Can you work these out from the model? Positions are in its coordinate system, mm. A direction names the side the tool comes from. Give positions to 0.01 mm unless a question says otherwise; leave off trailing zeros. Order: outer loops, then holes, each group sorted by start corner. A loop starts at its lowest first (then second) coordinate and runs counter-clockwise, first axis right, second up. Notation, with made-up numbers: (80, 52) - (129, 52) arc R22 cw to (129, 89) - close; hole circle Ø7 at (64, -15). An arc over 180 degrees is marked (long way). One line per question, with ' | ' between items.
```python
from build123d import *

# Parameters (mm, degrees)
SKETCH_1_R      = 1.5
EXTRUDE_1_DEPTH = 3


with BuildPart() as part:
    # 草图1 → 凸台-拉伸1 (new body)
    with BuildSketch(Plane.XY):
        with BuildLine():
            Line((-3, -336.18), (-3, -372.501331749))
            Line((-3, -372.501331749), (116, -372.501331749))
            Line((116, -372.501331749), (116, -336.18))
            ThreePointArc((116, -336.18), (118, -332.18), (116, -328.18))
            Line((116, -328.18), (116, -4))
            ThreePointArc((116, -4), (116.535533906, 3.535533906), (109, 3))
            Line((109, 3), (106, 3))
            Line((106, 3), (106, -21.645755349))
            Line((106, -21.645755349), (7, -21.645755349))
            Line((7, -21.645755349), (7, 3))
            Line((7, 3), (4, 3))
            ThreePointArc((4, 3), (-3.535533906, 3.535533906), (-3, -4))
            Line((-3, -4), (-3, -328.18))
            ThreePointArc((-3, -328.18), (-5, -332.18), (-3, -336.18))
        make_face()
        Circle(SKETCH_1_R, mode=Mode.SUBTRACT)
        with Locations((113, 0)):
            Circle(SKETCH_1_R, mode=Mode.SUBTRACT)
        with Locations((0, -332.18)):
            Circle(SKETCH_1_R, mode=Mode.SUBTRACT)
        with Locations((113, -332.18)):
            Circle(SKETCH_1_R, mode=Mode.SUBTRACT)
        with BuildLine():
            Line((11, -99.104501604), (11, -342.524894505))
            ThreePointArc((11, -342.524894505), (13.928932188, -349.595962317), (21, -352.524894505))
            Line((21, -352.524894505), (71.385479273, -352.524894505))
            ThreePointArc((71.385479273, -352.524894505), (79.263756472, -348.683851265), (81.089872995, -340.111444179))
            Line((81.089872995, -340.111444179), (20.846592628, -97.875461369))
            ThreePointArc((20.846592628, -97.875461369), (15.380711351, -94.143001673), (11, -99.104501604))
        make_face(mode=Mode.SUBTRACT)
        with BuildLine():
            Line((100.988154046, -37.00591772), (100.615591755, -351.791020996))
            ThreePointArc((100.615591755, -351.791020996), (97.985405334, -354.764589688), (94.70763828, -352.524894505))
            Line((94.70763828, -352.524894505), (15.005818776, -38.229040236))
            ThreePointArc((15.005818776, -38.229040236), (15.906197954, -33.929592957), (19.852411404, -32))
            Line((19.852411404, -32), (95.988157548, -32))
            ThreePointArc((95.988157548, -32), (99.525783065, -33.466558944), (100.988154046, -37.00591772))
        make_face(mode=Mode.SUBTRACT)
    extrude(amount=EXTRUDE_1_DEPTH)


solid = part.part
```
(1) Imagine slicing it at C-C (x = 86). List the corners of the cut face in (y, z) for me.
Answer below:
outline: (-372.5, 0) - (-318.19, 0) - (-318.19, 3) - (-372.5, 3) - close; (-32, 0) - (-21.65, 0) - (-21.65, 3) - (-32, 3) - close
(2) Imagine slicing it at B-B (y = -324.5). List the corners of the cut face in (x, z) for me.
Answer below:
outline: (-3, 0) - (11, 0) - (11, 3) - (-3, 3) - close; (77.21, 0) - (87.6, 0) - (87.6, 3) - (77.21, 3) - close; (100.65, 0) - (116, 0) - (116, 3) - (100.65, 3) - close
(3) On a 3-axis mill with a long thin cutter (end or side, diameter ignored), from which of +Z, -Z, +X, -X, +Y, -Y can I reach the whole of each face in a straight line? I mean faces 3 (the face through (52, -211, 0)), 4 (the face through (79.185, -348.783, 1.479)). Say none if no direction works.
Answer below:
face 3: -Z, +X, -X, +Y, -Y | face 4: +Z, -Z
(4) If we mould it in two halves opening along Y, with no side actions, what happens to faces 1 (the face through (51.39, -220.69, 1.48)), 2 (the face through (52, -211, 3))? For each: released by +Y, released by -Y, zero draft, split by the parting line, or undercut.
Answer below:
face 1: undercut | face 2: zero draft
(5) If I drill on line 1 (Y direction, x = 113, z = 1.6); line 2 (X direction, y = -248, z = 2.45); line 3 (X direction, y = -101.5, z = 2.4), over which ranges is the centre line in solid material (lowest first)?
Answer below:
line 1: -372.5 to -333.68, -330.68 to -1.5, 1.5 to 5 | line 2: -3 to 11, 58.18 to 68.2, 100.74 to 116 | line 3: -3 to 11, 21.75 to 31.05, 100.91 to 116
(6) Will these pins go through, and if not, where does the flat tip stop? pin 1 (1.5 mm diameter, centred on x = 107, z = 2, fed in from +Y); pin 2 (1.5 mm diameter, centred on y = -192, z = 1.5, fed in from +X); pin 3 (0.9 mm diameter, centred on y = -354.5, z = 1.5, fed in from -X).
Answer below:
pin 1: y = 3 | pin 2: x = 116 | pin 3: x = -3
(7) Imagine slicing it at D-D (x = 28). List the corners of the cut face in (y, z) for me, and give its area (3 significant figures).
Answer below:
outline: (-372.5, 0) - (-352.52, 0) - (-352.52, 3) - (-372.5, 3) - close; (-126.64, 0) - (-89.47, 0) - (-89.47, 3) - (-126.64, 3) - close; (-32, 0) - (-21.65, 0) - (-21.65, 3) - (-32, 3) - close | area: 202 mm^2
(8) Imagine slicing it at A-A (z = 2.45). Count the separate pieces of the cut face and the enclosed holes in it, and give its area (3 significant figures).
Answer below:
separate pieces: 1 | enclosed holes: 6 | area: 16,800 mm^2
